from build123d import *

# Parameters (mm, degrees)
F0_R     = 5.08
F1_DEPTH = 12.7
F0_W     = 6.35
F0_H     = 6.35
F0_R_2   = 1.905
F2_DEPTH = 25.4
F3_DEPTH = 63.5


with BuildPart() as f1:
    # F0 (on Top) → F1 (new body)
    with BuildSketch(Plane.XY):
        with BuildLine():
            ThreePointArc((-57.1493167461, -20.6207571715), (-68.9814302299, -26.9707571715), (-57.1493167461, -33.3207571715))
            ThreePointArc((-57.1493167461, -33.3207571715), (-54.6472398563, -30.5740955718), (-53.7414302299, -26.9707571715))
            ThreePointArc((-53.7414302299, -26.9707571715), (-54.6472398563, -23.3674187712), (-57.1493167461, -20.6207571715))
        make_face()
        with Locations((-61.3614302299, -26.9707571715)):
            Circle(F0_R, mode=Mode.SUBTRACT)
    extrude(amount=F1_DEPTH)

    # F0 (on Top) → F2 (join)
    with BuildSketch(Plane.XY):
        with BuildLine():
            Line((-53.7414302299, -26.9707571715), (-32.9907516612, -26.9707571715))
            Line((-32.9907516612, -26.9707571715), (-32.9907516612, -20.6207571715))
            Line((-32.9907516612, -20.6207571715), (-57.1493167461, -20.6207571715))
            ThreePointArc((-57.1493167461, -20.6207571715), (-54.6472398563, -23.3674187712), (-53.7414302299, -26.9707571715))
        make_face()
        with Locations((-23.4657516612, -23.7957571715)):
            Rectangle(F0_W, F0_H)
        with Locations((-23.4657516612, -23.7957571715)):
            Circle(F0_R_2, mode=Mode.SUBTRACT)
        with Locations((-29.8157516612, -23.7957571715)):
            Rectangle(F0_W, F0_H)
        with Locations((-29.8157516612, -23.7957571715)):
            Circle(F0_R_2, mode=Mode.SUBTRACT)
    extrude(amount=F2_DEPTH)

    # F0 (on Top) → F3 (join)
    with BuildSketch(Plane.XY):
        with BuildLine():
            Line((-53.7414302299, -26.9707571715), (-32.9907516612, -26.9707571715))
            Line((-32.9907516612, -26.9707571715), (-32.9907516612, -20.6207571715))
            Line((-32.9907516612, -20.6207571715), (-57.1493167461, -20.6207571715))
            ThreePointArc((-57.1493167461, -20.6207571715), (-54.6472398563, -23.3674187712), (-53.7414302299, -26.9707571715))
        make_face()
    extrude(amount=F3_DEPTH)

    # F4: F1 across face


with BuildPart() as f1_1:
    add(f1.part)
    add(f1.part.mirror(Plane(origin=(-43.8925069162, -23.7183782797, 63.5), x_dir=(1, 0, 0), z_dir=(0, 0, 1))))


solid = f1_1.part
Here's how the part is built. I have some questions about the finished solid (model axes, mm). A direction names the side the tool comes from. Round coordinates to 2 decimals unless told otherwise and drop trailing zeros. Loops run counter-clockwise (first coordinate to the right, second up) from the corner with the lowest first, then second, coordinate; pieces in that order, holes last.
1. For P1, Ø12, axis at x = -39.5, z = 71, coming from the -Y side; P2, Ø10, axis at x = -51, z = 13, coming from the -Y side; P3, Ø3, axis at y = -24.5, z = 51.5, coming from the +X side, each with a flat end and sliding along its axis, tell me the tip position at first contact or that it passes through.
Answer list:
P1: stops at y = -26.97
P2: stops at y = -32.38
P3: stops at x = -32.99
2. If we section it at B-B on y = -29.5: Write out the boundary of the cut face in (x, z).
Answer list:
outline: (-68.55, 0) - (-65.77, 0) - (-65.77, 12.7) - (-68.55, 12.7) - close; (-68.55, 114.3) - (-65.77, 114.3) - (-65.77, 127) - (-68.55, 127) - close; (-56.96, 0) - (-54.17, 0) - (-54.17, 12.7) - (-56.96, 12.7) - close; (-56.96, 114.3) - (-54.17, 114.3) - (-54.17, 127) - (-56.96, 127) - close
3. If we section it at D-D on z = 50.5: Write out the boundary of the cut face in (x, y).
Answer list:
outline: (-57.15, -20.62) arc R7.62 cw to (-53.74, -26.97) - (-32.99, -26.97) - (-32.99, -20.62) - close
4. We'd pull the mould along X, two halves only. Please class faces 1 (the face through (-20.291, -24, 114)), 2 (the face through (-50, -25, 0)), 3 (the face through (-66.437, -26.747, 6.261)): +X half, -X half, draft (parallel to the pull), parting line (faces both ways), or undercut.
Answer list:
face 1: +X half
face 2: draft
face 3: undercut
5. If I drill on line 1 along Y through (x, z) = (-23.5, 20.5); line 2 along X through (y, z) = (-23, 8); line 3 along Z through (x, y) = (-64.5, -33.5), over which ranges is the centre line in solid material (lowest first)?
Answer list:
line 1: y = -26.97 to -25.7, -21.89 to -20.62
line 2: x = -67.87 to -64.53, -58.19 to -31.55, -28.08 to -25.2, -21.73 to -20.29
line 3: z = 0 to 12.7, 114.3 to 127
6. If we section it at C-C on z = 117: Write out the boundary of the cut face in (x, y) (3 decimals), plus the area to 3 significant figures.
Answer list:
outline: (-57.149, -20.621) arc R7.62 ccw (long way) to (-53.741, -26.971) - (-20.291, -26.971) - (-20.291, -20.621) - close; hole circle Ø10.16 at (-61.361, -26.971); hole circle Ø3.81 at (-29.816, -23.796); hole circle Ø3.81 at (-23.466, -23.796)
area: 297 mm2
7. If we section it at A-A on x = -59: Write out the boundary of the cut face in (y, z), plus the area to 3 significant figures.
Answer list:
outline: (-34.22, 0) - (-31.47, 0) - (-31.47, 12.7) - (-34.22, 12.7) - close; (-34.22, 114.3) - (-31.47, 114.3) - (-31.47, 127) - (-34.22, 127) - close; (-22.47, 0) - (-19.73, 0) - (-19.73, 12.7) - (-22.47, 12.7) - close; (-22.47, 114.3) - (-19.73, 114.3) - (-19.73, 127) - (-22.47, 127) - close
area: 140 mm2
8. Which directions (+Z, -Z, +X, -X, +Y, -Y) give clear straight access to the entire face, cutting with the end or side of a thin tool? Please do faces 4 (the face through (-27, -24, 101.6)), 5 (the face through (-41, -26.971, 64)), 6 (the face through (-56, -29, 12.7)).
Answer list:
face 4: +X, +Y, -Y
face 5: +Z, -Z, +X, -Y
face 6: -X, -Y
